Source: CAD feature listing. Evaluate the final solid. Frame: model axes, mm. Face numbers are marked on the shaded views. A direction names the side the tool comes from. Coordinates: 2 decimals unless noted, no trailing zeros. Order: outer loops, then holes, each group sorted by start corner. A loop starts at its lowest first (then second) coordinate and runs counter-clockwise, first axis right, second up. Notation, with made-up numbers: (8.5, 40) -> (49.5, 40) arc R10 cw to (49.5, 50) -> close; hole circle Ø2 at (-31.5, 54.5). An arc over 180 degrees is marked (long way). Write item = value, one per line. Start each with the question number.
Item 1: Mould query, pull axis X, two halves, no side actions, for the marked faces 4, 5 and 6. Classes: released by +X, released by -X, zero draft, split by the parting line, or undercut.
Item 2: Contact query for flat-ended pins moving along their axis: pin 1 (0.8 mm diameter, centred on x = 50, y = -0.5, fed in from -Z); pin 2 (3 mm diameter, centred on x = 8, z = -39.5, fed in from -Y); pin 3 (1.5 mm diameter, centred on y = 10, z = -20, fed in from -X). Output: stop coordinate, or through.
Item 3: Ray query, line 1 along X through (y, z) = (8.25, -35.5); line 2 along X through (y, z) = (6, -37); line 3 along Y through (x, z) = (29.5, -48). Return the intervals inside material, ascending. Write a range as [from, to].
Item 4: Section query C-C (x = 39). Output: boundary loops of the cut face in (y, z).
Item 5: Section query D-D (z = -17.5). Output: boundary loops of the cut face in (x, y).
Item 6: Section query A-A (z = -38.5). Output: boundary loops of the cut face in (x, y).
Item 7: Section query B-B (y = 8.75). Output: boundary loops of the cut face in (x, z), then the cut area to 3 significant figures.
Item 8: Set-up query: the marked faces 1, 2 and 3. Return all of +Z, -Z, +X, -X, +Y, -Y with unobstructed straight access to the full face (end or side cutting, diameter ignored); none if empty.
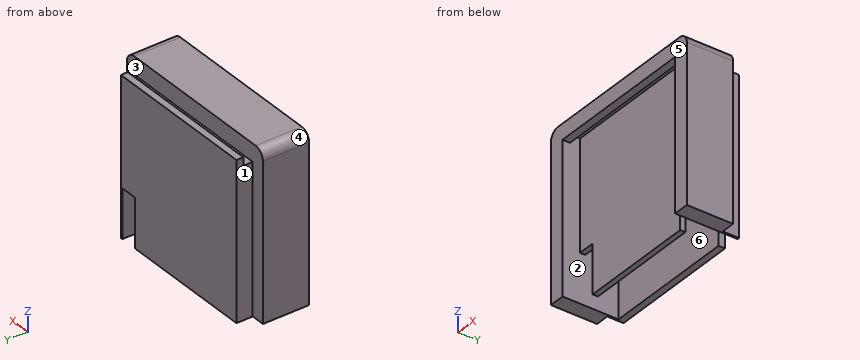
```python
from build123d import *

# Parameters (mm, degrees)
BOSS_EXTRUDE8_DEPTH  = 10.2
SKETCH8_W            = 56
SKETCH8_H            = 51
BOSS_EXTRUDE9_DEPTH  = 2
CUT_EXTRUDE1_START   = -4
CUT_EXTRUDE1_DEPTH   = 48
SKETCH12_W           = 4
SKETCH12_H           = 51
CUT_EXTRUDE2_DEPTH   = 5
SKETCH11_W           = 56
SKETCH11_H           = 2
BOSS_EXTRUDE10_DEPTH = 51
SKETCH11_3_W         = 56
SKETCH11_3_H         = 2.5
BOSS_EXTRUDE11_DEPTH = 2.5
SKETCH11_4_W         = 56
SKETCH11_4_H         = 2.5
BOSS_EXTRUDE12_DEPTH = 5
SKETCH13_W           = 5
SKETCH13_H           = 48.5
BOSS_EXTRUDE13_DEPTH = 5
SKETCH14_W           = 5
SKETCH14_H           = 14.2
SKETCH14_H_2         = 7
CUT_EXTRUDE3_DEPTH   = 15
FILLET1_R            = 3
MOVE_FACE1_BY        = 0.2
MOVE_FACE1_2_BY      = 0.2
MOVE_FACE1_3_BY      = 0.2
MOVE_FACE1_4_BY      = 0.2
MOVE_FACE2_BY        = 0.2
MOVE_FACE2_2_BY      = 0.2
MOVE_FACE2_3_BY      = 0.2
MOVE_FACE2_4_BY      = 0.2
MOVE_FACE2_5_BY      = 0.2
MOVE_FACE3_BY        = 0.2
MOVE_FACE3_2_BY      = 0.2
MOVE_FACE3_3_BY      = 0.2
MOVE_FACE3_4_BY      = 0.2
MOVE_FACE3_5_BY      = 0.2
MOVE_FACE3_6_BY      = 0.2


with BuildPart() as part:
    # Sketch1 → Boss-Extrude8 (new body)
    with BuildSketch(Plane(origin=(0, 0, 0), x_dir=(1, 0, 0), z_dir=(0, 1, 0))):
        Polygon((0, 51), (5, 51), (5, 49), (5, 7), (51, 7), (51, 51), (56, 51), (56, 0), (0, 0), align=None)
    extrude(amount=BOSS_EXTRUDE8_DEPTH)

    # Sketch8 → Boss-Extrude9 (add)
    with BuildSketch(Plane(origin=(0, 10.2, 0), x_dir=(1, 0, 0), z_dir=(0, 1, 0))):
        with Locations((28, 25.5)):
            Rectangle(SKETCH8_W, SKETCH8_H)
    extrude(amount=BOSS_EXTRUDE9_DEPTH)

    # Sketch10 → Cut-Extrude1 (cut)
    with BuildSketch(Plane.ZY.offset(CUT_EXTRUDE1_START)):
        Polygon((0, 12.2), (-2.5, 12.2), (-2.5, 9.7), (-5, 9.7), (-5, 7.2), (0, 7.2), align=None)
    extrude(amount=-CUT_EXTRUDE1_DEPTH, mode=Mode.SUBTRACT)

    # Sketch12 → Cut-Extrude2 (cut)
    with BuildSketch(Plane(origin=(0, 12.2, 0), x_dir=(1, 0, 0), z_dir=(0, 1, 0))):
        with Locations((2, 25.5)):
            Rectangle(SKETCH12_W, SKETCH12_H)
        with Locations((54, 25.5)):
            Rectangle(SKETCH12_W, SKETCH12_H)
    extrude(amount=-CUT_EXTRUDE2_DEPTH, mode=Mode.SUBTRACT)

    # Sketch11 → Boss-Extrude10 (add)
    with BuildSketch(Plane.XY):
        with Locations((28, -1)):
            Rectangle(SKETCH11_W, SKETCH11_H)
    extrude(amount=-BOSS_EXTRUDE10_DEPTH)

    # Sketch11<3> → Boss-Extrude11 (add)
    with BuildSketch(Plane.XY):
        with Locations((28, -3.25)):
            Rectangle(SKETCH11_3_W, SKETCH11_3_H)
    extrude(amount=-BOSS_EXTRUDE11_DEPTH)

    # Sketch11<4> → Boss-Extrude12 (add)
    with BuildSketch(Plane.XY):
        with Locations((28, -5.75)):
            Rectangle(SKETCH11_4_W, SKETCH11_4_H)
    extrude(amount=-BOSS_EXTRUDE12_DEPTH)

    # Sketch13 → Boss-Extrude13 (add)
    with BuildSketch(Plane.XZ.offset(2)):
        with Locations((2.5, -26.75)):
            Rectangle(SKETCH13_W, SKETCH13_H)
        with Locations((53.5, -26.75)):
            Rectangle(SKETCH13_W, SKETCH13_H)
    extrude(amount=BOSS_EXTRUDE13_DEPTH)

    # Sketch14 → Cut-Extrude3 (cut)
    with BuildSketch(Plane(origin=(0, 0, -51), x_dir=(-1, 0, 0), z_dir=(0, 0, -1))):
        with Locations((-48.5, 5.1)):
            Rectangle(SKETCH14_W, SKETCH14_H)
        with Locations((-7.5, -3.5)):
            Rectangle(SKETCH14_W, SKETCH14_H_2)
    extrude(amount=-CUT_EXTRUDE3_DEPTH, mode=Mode.SUBTRACT)

    # Fillet1
    fillet1_edges = [part.edges().sort_by_distance(p)[0] for p in [
        (56, 0.1, 0),
        (0, 0.1, 0),
    ]]
    fillet(fillet1_edges, radius=FILLET1_R)

    # Move Face1: a face moved inward by 0.2
    extrude(part.faces().sort_by_distance((28, 9.7, -3.75))[0], amount=MOVE_FACE1_BY, dir=(0, 1, 0), mode=Mode.SUBTRACT)

    # Move Face1 2: a face moved inward by 0.2
    extrude(part.faces().sort_by_distance((28, 10.95, -2.5))[0], amount=MOVE_FACE1_2_BY, dir=(0, 0, -1), mode=Mode.SUBTRACT)

    # Move Face1 3: a face moved inward by 0.2
    extrude(part.faces().sort_by_distance((28, 8.45, -5))[0], amount=MOVE_FACE1_3_BY, dir=(0, 0, -1), mode=Mode.SUBTRACT)

    # Move Face1 4: a face moved inward by 0.2
    extrude(part.faces().sort_by_distance((28, -2, -25.542647765))[0], amount=MOVE_FACE1_4_BY, dir=(0, 1, 0), mode=Mode.SUBTRACT)

    # Move Face2: a face moved inward by 0.2
    extrude(part.faces().sort_by_distance((28, 9.9, -3.95))[0], amount=MOVE_FACE2_BY, dir=(0, 1, 0), mode=Mode.SUBTRACT)

    # Move Face2 2: a face moved inward by 0.2
    extrude(part.faces().sort_by_distance((28, 8.55, -5.2))[0], amount=MOVE_FACE2_2_BY, dir=(0, 0, -1), mode=Mode.SUBTRACT)

    # Move Face2 3: a face moved inward by 0.2
    extrude(part.faces().sort_by_distance((28, 11.05, -2.7))[0], amount=MOVE_FACE2_3_BY, dir=(0, 0, -1), mode=Mode.SUBTRACT)

    # Move Face2 4: a face moved inward by 0.2
    extrude(part.faces().sort_by_distance((52, 9.733067093, -27.508466454))[0], amount=MOVE_FACE2_4_BY, dir=(-1, 0, 0), mode=Mode.SUBTRACT)

    # Move Face2 5: a face moved inward by 0.2
    extrude(part.faces().sort_by_distance((4, 9.733067093, -27.508466454))[0], amount=MOVE_FACE2_5_BY, dir=(1, 0, 0), mode=Mode.SUBTRACT)

    # Move Face3: a face moved inward by 0.2
    extrude(part.faces().sort_by_distance((5, 1.649930724, -28.974870107))[0], amount=MOVE_FACE3_BY, dir=(-1, 0, 0), mode=Mode.SUBTRACT)

    # Move Face3 2: a face moved inward by 0.2
    extrude(part.faces().sort_by_distance((51, 2.03104423, -29.55452278))[0], amount=MOVE_FACE3_2_BY, dir=(1, 0, 0), mode=Mode.SUBTRACT)

    # Move Face3 3: a face moved inward by 0.2
    extrude(part.faces().sort_by_distance((28, -5.75, -5))[0], amount=MOVE_FACE3_3_BY, dir=(0, 0, 1), mode=Mode.SUBTRACT)

    # Move Face3 4: a face moved inward by 0.2
    extrude(part.faces().sort_by_distance((28, -4.5, -3.75))[0], amount=MOVE_FACE3_4_BY, dir=(0, -1, 0), mode=Mode.SUBTRACT)

    # Move Face3 5: a face moved inward by 0.2
    extrude(part.faces().sort_by_distance((28, -3.15, -2.5))[0], amount=MOVE_FACE3_5_BY, dir=(0, 0, 1), mode=Mode.SUBTRACT)

    # Move Face3 6: a face moved inward by 0.2
    extrude(part.faces().sort_by_distance((28, -1.8, -25.542647765))[0], amount=MOVE_FACE3_6_BY, dir=(0, 1, 0), mode=Mode.SUBTRACT)


solid = part.part
```
Computed:
q1.face_4 = released by -X
q1.face_5 = zero draft
q1.face_6 = undercut
q2.pin_1 = -36
q2.pin_2 = 10.2
q2.pin_3 = 4.2
q3.line_1 = [4.2, 4.8], [51.2, 51.8]
q3.line_2 = [0, 4.8], [51.2, 56]
q3.line_3 = [-1.6, 0], [10.2, 12.2]
q4.outline = (-7, -4.8) -> (-4.7, -4.8) -> (-4.7, -2.3) -> (-1.6, -2.3) -> (-1.6, -51) -> (0, -51) -> (0, -7) -> (10.2, -7) -> (10.2, -51) -> (12.2, -51) -> (12.2, -2.9) -> (10.1, -2.9) -> (10.1, -5.4) -> (7.2, -5.4) -> (7.2, 0) -> (-7, 0) -> close
q5.outline = (0, -7) -> (4.8, -7) -> (4.8, -1.6) -> (51.2, -1.6) -> (51.2, -7) -> (56, -7) -> (56, 7.2) -> (51.8, 7.2) -> (51.8, 12.2) -> (4.2, 12.2) -> (4.2, 7.2) -> (0, 7.2) -> close; hole (4.8, 0) -> (51.2, 0) -> (51.2, 10.2) -> (4.8, 10.2) -> close
q6.outline = (0, -7) -> (4.8, -7) -> (4.8, 10.2) -> (46, 10.2) -> (46, 12.2) -> (4.2, 12.2) -> (4.2, 7.2) -> (0, 7.2) -> close; (10, -1.6) -> (46, -1.6) -> (46, 0) -> (10, 0) -> close; (51.2, -7) -> (56, -7) -> (56, 7.2) -> (51.8, 7.2) -> (51.8, 12.2) -> (51.2, 12.2) -> close
q7.outline = (4.2, -51) -> (4.8, -51) -> (4.8, -7) -> (51.2, -7) -> (51.2, -51) -> (51.8, -51) -> (51.8, -5.4) -> (4.2, -5.4) -> close
q7.area = 129 mm^2
q8.face_1 = +Z, -Z, -X, +Y
q8.face_2 = -Z
q8.face_3 = +Z
